Input: part model. Units: mm. Frame: model coordinates. A direction names the side the tool comes from. Give positions to 0.01 mm unless a question says otherwise; leave off trailing zeros. Loops run counter-clockwise (first coordinate to the right, second up) from the corner with the lowest first, then second, coordinate; pieces in that order, holes last. Notation, with made-up numbers: M 82.25,-19.5 L 130.25,-19.5 A15 cw 130.25,4.5 Z; hole C -14,25.25 d7. An arc over 180 degrees is marked long. One line per item, written item: value. Start each with the question number.
(1) Pull-direction query (X, two-part tool) for faces 6 (the flat face through (-30.6, 0, 3)), 7 (the cylindrical face through (-24.17, 33.59, 2.99)), 8 (the flat face through (29, -34, 3)), 9 (the flat face through (20.164, 30.281, 4.986)); classes: released by +X, released by -X, zero draft, split by the parting line, or undercut.
(2) Ray query, line 1 along Y through (x, z) = (21.5, 3); line 2 along Y through (x, z) = (5.5, 0.75); line 3 along X through (y, z) = (31, 4.25). Return the intervals inside material, ascending. Write a range as from..to.
(3) Section A-A on x = -7.5. Output: boundary loops of the cut face in (y, z).
(4) Section D-D on x = 20.5. Output: boundary loops of the cut face in (y, z), plus the area to 3 significant figures.
(5) Section B-B on z = 4.75. Output: boundary loops of the cut face in (x, y) (3 decimals), plus the area to 3 significant figures.
(6) Section C-C on z = 1. Output: boundary loops of the cut face in (x, y).
(7) Access query for faces 1 (the flat face through (-20.164, -30.281, 1.014)), 2 (the flat face through (20.164, 30.281, 1.014)), 3 (the cylindrical face through (-15.204, -28.676, 2.986)), 4 (the conical face through (15.406, 27.707, 4.986)), 5 (the cylindrical face through (24.088, 33.564, 2.986)). Directions: +Z, -Z, +X, -X, +Y, -Y. A direction counts if a zero-diameter tool reaches every point of the face in a straight line with its end or side. Return the directions, or none.
(8) Pin query (flat end, axial travel): P1, Ø1, axis at x = -23, z = 4.5, coming from the -Y side; P2, Ø0.6, axis at x = 0, z = 3, coming from the +Y side; P3, Ø2, axis at x = 1.5, z = 3, coming from the -Y side. Return the tip coordinate at first contact, or that it passes through.
```python
from build123d import *

# Parameters (mm, degrees)
CROQUIS1_W              = 61.2
CROQUIS1_H              = 68
SALIENTE_EXTRUIR1_DEPTH = 6
CORTAR_EXTRUIR1_DEPTH   = 47.134152209
REDONDEO1_R             = 10
CHAFL_N1_SIZE           = 2


with BuildPart() as part:
    # Croquis1 → Saliente-Extruir1 (new body)
    with BuildSketch(Plane.XY):
        Rectangle(CROQUIS1_W, CROQUIS1_H)
    extrude(amount=SALIENTE_EXTRUIR1_DEPTH)

    # Croquis2 → Cortar-Extruir1 (cut, through all)
    with BuildSketch(Plane.XY.offset(6)):
        Polygon((-24, 34), (-15.292264831, 28.240639048), (15.292264831, 28.240639048), (24, 34), align=None)
        Polygon((24, -34), (15.292264831, -28.240639048), (-15.292264831, -28.240639048), (-24, -34), align=None)
    extrude(amount=-CORTAR_EXTRUIR1_DEPTH, mode=Mode.SUBTRACT)

    # Redondeo1
    redondeo1_edges = [part.edges().sort_by_distance(p)[0] for p in [
        (-24, 34, 3),
        (24, 34, 3),
        (15.292264831, 28.240639048, 3),
        (-15.292264831, 28.240639048, 3),
        (24, -34, 3),
        (-24, -34, 3),
        (-15.292264831, -28.240639048, 3),
        (15.292264831, -28.240639048, 3),
    ]]
    fillet(redondeo1_edges, radius=REDONDEO1_R)

    # Chaflán1
    chafl_n1_edges = [part.edges().sort_by_distance(p)[0] for p in [
        (28.803922608, 34, 6),
        (19.646132416, -31.120319524, 6),
        (19.646132416, -31.120319524, 0),
        (19.646132416, 31.120319524, 6),
        (0, 28.240639048, 6),
        (28.803922608, 34, 0),
        (-19.646132416, 31.120319524, 6),
        (-28.803922608, 34, 6),
        (-19.646132416, -31.120319524, 6),
        (0, -28.240639048, 6),
        (28.803922608, -34, 6),
        (-24.127474692, 33.576192648, 6),
        (24.127474692, 33.576192648, 6),
        (-24.127474692, -33.576192648, 6),
        (24.127474692, -33.576192648, 6),
        (28.803922608, -34, 0),
        (0, 28.240639048, 0),
        (19.646132416, 31.120319524, 0),
        (0, -28.240639048, 0),
        (-28.803922608, -34, 0),
        (-19.646132416, -31.120319524, 0),
        (-28.803922608, 34, 0),
        (-19.646132416, 31.120319524, 0),
        (-24.127474692, 33.576192648, 0),
        (24.127474692, 33.576192648, 0),
        (-24.127474692, -33.576192648, 0),
        (24.127474692, -33.576192648, 0),
        (15.164790139, -28.6644464, 6),
        (15.164790139, -28.6644464, 0),
        (-15.164790139, -28.6644464, 6),
        (-15.164790139, -28.6644464, 0),
        (15.164790139, 28.6644464, 6),
        (15.164790139, 28.6644464, 0),
        (-15.164790139, 28.6644464, 6),
        (-15.164790139, 28.6644464, 0),
        (-28.803922608, -34, 6),
    ]]
    chamfer(chafl_n1_edges, length=CHAFL_N1_SIZE)


solid = part.part
```
Output values:
1. face 6: released by -X
1. face 7: undercut
1. face 8: zero draft
1. face 9: undercut
2. line 1: y = -32.35..32.35
2. line 2: y = -26.99..26.99
2. line 3: x = -30.6..-19.92, 19.92..30.6
3. outline: M -28.24,2 L -26.24,0 L 26.24,0 L 28.24,2 L 28.24,4 L 26.24,6 L -26.24,6 L -28.24,4 Z
4. outline: M -31.69,2 L -29.29,0 L 29.29,0 L 31.69,2 L 31.69,4 L 29.29,6 L -29.29,6 L -31.69,4 Z
4. area: 371 mm²
5. outline: M -30.6,-33.25 L -27.008,-33.25 A9.25 ccw -21.905,-31.715 L -18.215,-29.274 A10.75 cw -12.284,-27.491 L 12.284,-27.491 A10.75 cw 18.215,-29.274 L 21.905,-31.715 A9.25 ccw 27.008,-33.25 L 30.6,-33.25 L 30.6,33.25 L 27.008,33.25 A9.25 ccw 21.905,31.715 L 18.215,29.274 A10.75 cw 12.284,27.491 L -12.284,27.491 A10.75 cw -18.215,29.274 L -21.905,31.715 A9.25 ccw -27.008,33.25 L -30.6,33.25 Z
5. area: 3,610 mm²
6. outline: M -30.6,-33 L -27.01,-33 A9 ccw -22.04,-31.51 L -18.35,-29.07 A11 cw -12.28,-27.24 L 12.28,-27.24 A11 cw 18.35,-29.07 L 22.04,-31.51 A9 ccw 27.01,-33 L 30.6,-33 L 30.6,33 L 27.01,33 A9 ccw 22.04,31.51 L 18.35,29.07 A11 cw 12.28,27.24 L -12.28,27.24 A11 cw -18.35,29.07 L -22.04,31.51 A9 ccw -27.01,33 L -30.6,33 Z
7. face 1: -Z, -Y
7. face 2: -Z, +Y
7. face 3: +Z, -Z, -Y
7. face 4: +Z, +Y
7. face 5: +Z, -Z, +Y
8. P1: stops at y = -33.2
8. P2: stops at y = 28.24
8. P3: stops at y = -28.24
